Source: CAD feature listing. Evaluate the final solid. Frame: model axes, mm. A direction names the side the tool comes from. Give positions to 0.01 mm unless a question says otherwise; leave off trailing zeros. Write each loop counter-clockwise with the first axis right and the second up, starting at its lowest first coordinate (ties: lowest second). Pieces come first, ordered by that corner, then holes. Notation, with made-up numbers: (-1.75, 55) -> (31.25, 55) arc R25 cw to (31.25, 75) -> close; hole circle Ø1 at (-0.5, 39.25). An arc over 180 degrees is marked (long way). Use one line per item in the form item = value. Start each with the question number.
(1) Material intervals for line 1 along Y through (x, z) = (-55, 4); line 2 along X through (y, z) = (30, 2.5); line 3 along Y through (x, z) = (-5.5, 6.75), sorted ascending. Write a range as from..to.
(2) Set-up query: faces 1 (the face through (-55.07, -31.6, 4.06)), 2 (the face through (-50, -1, 9)), 3 (the face through (-10, 1, 9)). Return all of +Z, -Z, +X, -X, +Y, -Y with unobstructed straight access to the full face (end or side cutting, diameter ignored); none if empty.
(3) Draft query along X for faces 4 (the face through (-60, 1, 4)), 5 (the face through (0, -1, 4)), 6 (the face through (-35.495, 21.742, 5.07)). Return one class per face: pulls with the +X half, pulls with the -X half, needs draft (parallel to the pull), parting line crosses it, or undercut.
(4) Cut plane A-A, the plane x = -38. Output: boundary loops of the cut face in (y, z).
(5) Cut plane D-D, the plane z = 9. Count the separate pieces of the cut face and the enclosed holes in it, and give its area (3 significant figures).
(6) First-contact query: P1, Ø5, axis at x = -5, y = 30, coming from the +Z side; P2, Ø3, axis at x = -5, y = -30, coming from the +Z side; P3, Ø0.6, axis at y = 18, z = 9, coming from the -X side. Flat tips, straight axial feed; report the tip coordinate or a pass-through.
(7) Cut plane B-B, the plane y = 10.5. Output: boundary loops of the cut face in (x, z).
(8) Cut plane C-C, the plane y = 2. Output: boundary loops of the cut face in (x, z), and give its area (3 significant figures).
Solid Edge part; units mm, degrees
sketch "Sketch1" plane through (0, 0, 0) normal (0, 0, 1) x (1, 0, 0)
  line L0 (0, 40) -> (-100, 40)
  line L1 (-100, 40) -> (-100, -40)
  line L2 (-100, -40) -> (0, -40)
  line L3 (0, -40) -> (0, 40)
extrude "Protrusion1" add sketch "Sketch1" along normal blind 10
sketch "Sketch2" plane through (-30, 0, 10) normal (0, 0, 1) x (1, 0, 0)
  circle A0 centre (0, 21.5) radius 5.5
  circle A1 centre (0, -21.5) radius 5.5
extrude "Cutout1" cut sketch "Sketch2" against normal through all
sketch "Sketch3" plane through (-40, 0, 10) normal (0, 0, 1) x (1, 0, 0)
  circle A0 centre (10, 32.5) radius 1
  circle A1 centre (-1, 21.5) radius 1
  circle A2 centre (10, 10.5) radius 1
  circle A3 centre (21, 21.5) radius 1
  dimension "D1" = 10
extrude "Cutout2" cut sketch "Sketch3" against normal through all
sketch "Sketch4" plane through (-40, 0, 10) normal (0, 0, 1) x (1, 0, 0)
  circle A0 centre (2, -21.3736) radius 1
  circle A1 centre (10, -13.3736) radius 1
  circle A2 centre (18, -21.3736) radius 1
  circle A3 centre (10, -29.3736) radius 1
extrude "Cutout3" cut sketch "Sketch4" against normal through all
sketch "Sketch5" plane through (-40, 0, 10) normal (0, 0, 1) x (1, 0, 0)
  line L0 (40, 40) -> (30, 40)
  line L1 (30, 40) -> (30, -40)
  line L2 (30, -40) -> (40, -40)
  line L3 (40, -40) -> (40, 40)
extrude "Extrusionsausschnitt_4" cut sketch "Sketch5" against normal blind 2
sketch "Sketch6" plane through (-5, 0, 8) normal (0, 0, 1) x (0, 1, 0)
  circle A0 centre (-30, 0) radius 1.6
  circle A1 centre (30, 0) radius 1.6
  dimension "D1" = 30
extrude "Cutout4" cut sketch "Sketch6" against normal through all
sketch "Sketch7" plane through (-55, 0, 10) normal (0, 0, 1) x (0, -1, 0)
  line L0 (40, -45) -> (-40, -45)
  line L1 (-40, -45) -> (-40, -5)
  line L2 (-40, -5) -> (40, -5)
  line L3 (40, -5) -> (40, -45)
extrude "Cutout5" cut sketch "Sketch7" against normal through all
mirror "Mirror1" about plane through (-30, 0, 0) normal (1, 0, 0) of "Cutout4", "Extrusionsausschnitt_4"
properties material "Nylon, allgemein"
Geometry says:
q1.line_1 = -40..-31.6, -28.4..28.4, 31.6..40
q1.line_2 = -60..-56.6, -53.4..-6.6, -3.4..0
q1.line_3 = -40..-31.52, -28.48..28.48, 31.52..40
q2.face_1 = +Z, -Z
q2.face_2 = +Z, -X, +Y, -Y
q2.face_3 = +Z, +X, +Y, -Y
q3.face_4 = pulls with the -X half
q3.face_5 = pulls with the +X half
q3.face_6 = undercut
q4.outline = (-40, 0) -> (-22.37, 0) -> (-22.37, 10) -> (-40, 10) -> close; (-20.37, 0) -> (40, 0) -> (40, 10) -> (-20.37, 10) -> close
q5.separate_pieces = 1
q5.enclosed_holes = 10
q5.area = 2,980 mm^2
q6.P1 = 8
q6.P2 = through
q6.P3 = -50
q7.outline = (-60, 0) -> (-31, 0) -> (-31, 10) -> (-50, 10) -> (-50, 8) -> (-60, 8) -> close; (-29, 0) -> (0, 0) -> (0, 8) -> (-10, 8) -> (-10, 10) -> (-29, 10) -> close
q8.outline = (-60, 0) -> (0, 0) -> (0, 8) -> (-10, 8) -> (-10, 10) -> (-50, 10) -> (-50, 8) -> (-60, 8) -> close
q8.area = 560 mm^2
